Source: three-view drawing plus pictorial views. Frame: mm from the lowest corner of the part. Give positions to 0.01 mm unless a question says otherwise; leave off trailing zeros. Loops run counter-clockwise (first coordinate to the right, second up) from the corner with the lowest first, then second, coordinate; pieces in that order, holes last.
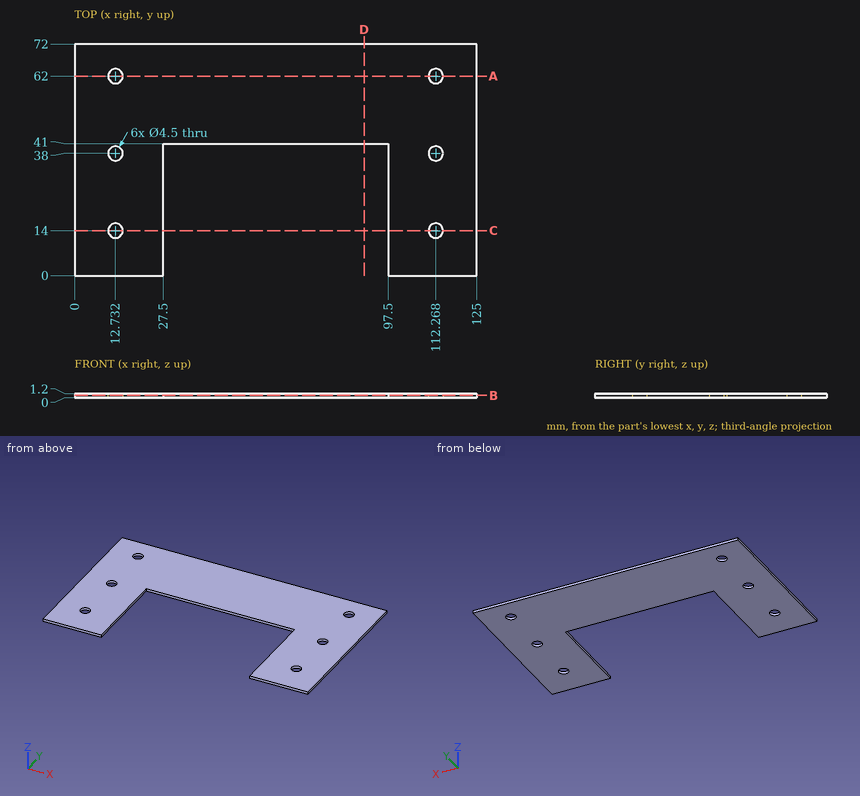
(1) Cut plane B-B (z = 0.65). Return the cut outline in (x, y).
Values follow:
outline: (0, 0) - (27.5, 0) - (27.5, 41) - (97.5, 41) - (97.5, 0) - (125, 0) - (125, 72) - (0, 72) - close; hole circle Ø4.5 at (12.73, 14); hole circle Ø4.5 at (12.73, 38); hole circle Ø4.5 at (12.73, 62); hole circle Ø4.5 at (112.27, 14); hole circle Ø4.5 at (112.27, 38); hole circle Ø4.5 at (112.27, 62)
(2) Ray query, probe 1 along X at (y, z) = (26.5, 0.2); probe 2 along Y at (x, z) = (112.5, 1.05); probe 3 along Y at (x, z) = (59, 0.6). Return the intervals inside material, ascending.
Values follow:
probe 1: x = 0 to 27.5, 97.5 to 125
probe 2: y = 0 to 11.76, 16.24 to 35.76, 40.24 to 59.76, 64.24 to 72
probe 3: y = 41 to 72
(3) Cut plane A-A (y = 62). Return the cut outline in (x, z).
Values follow:
outline: (0, 0) - (10.48, 0) - (10.48, 1.2) - (0, 1.2) - close; (14.98, 0) - (110.02, 0) - (110.02, 1.2) - (14.98, 1.2) - close; (114.52, 0) - (125, 0) - (125, 1.2) - (114.52, 1.2) - close
(4) Cut plane D-D (x = 90). Return the cut outline in (y, z), and give its area (3 significant figures).
Values follow:
outline: (41, 0) - (72, 0) - (72, 1.2) - (41, 1.2) - close
area: 37.2 mm2
(5) Cut plane C-C (y = 14). Return the cut outline in (x, z).
Values follow:
outline: (0, 0) - (10.48, 0) - (10.48, 1.2) - (0, 1.2) - close; (14.98, 0) - (27.5, 0) - (27.5, 1.2) - (14.98, 1.2) - close; (97.5, 0) - (110.02, 0) - (110.02, 1.2) - (97.5, 1.2) - close; (114.52, 0) - (125, 0) - (125, 1.2) - (114.52, 1.2) - close
